CAD build for the part. Positions are in the model's coordinates, mm. Round coordinates to 2 decimals unless told otherwise and drop trailing zeros. Order: outer loops, then holes, each group sorted by start corner. A loop starts at its lowest first (then second) coordinate and runs counter-clockwise, first axis right, second up. Notation, with made-up numbers: M 8.5,73 L 34.5,73 A19 ccw 34.5,86 Z; hole C -4,-17.5 d10. An arc over 180 degrees is marked long. Answer as a JSON object with one key per item and string values.
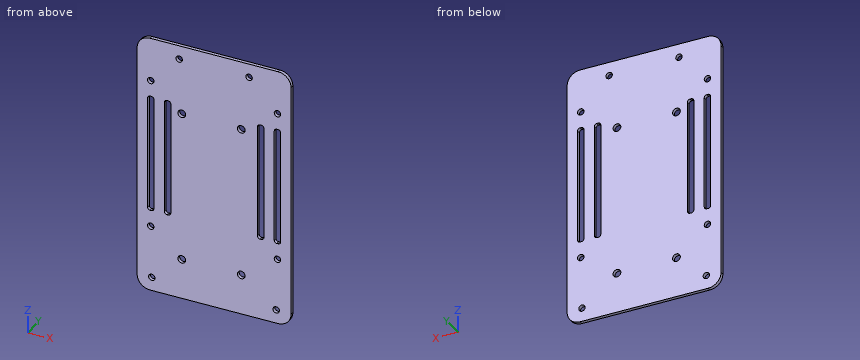
```python
from build123d import *

# Parameters (mm, degrees)
SKETCH2_W           = 59.5
SKETCH2_H           = 100.3
SKETCH2_R           = 1.25
SKETCH2_R_2         = 1.5
BOSS_EXTRUDE1_DEPTH = 1.35
FILLET1_R           = 5
CUT_EXTRUDE1_REACH  = 64.853
SKETCH3_W           = 2.5
SKETCH3_H           = 45.5
FILLET2_R           = 1


with BuildPart() as part:
    # Sketch2 → Boss-Extrude1 (new body)
    with BuildSketch(Plane(origin=(0, 0, 0), x_dir=(1, 0, 0), z_dir=(0, 1, 0))):
        with Locations((0, 5.2)):
            Rectangle(SKETCH2_W, SKETCH2_H)
        with Locations(Location((-24.5, 29.84, 0), (0, 0, 90))):
            Circle(SKETCH2_R, mode=Mode.SUBTRACT)
        with Locations(Location((-24.085, 50.1, 0), (0, 0, 90))):
            Circle(SKETCH2_R, mode=Mode.SUBTRACT)
        with Locations(Location((24.015, 50.1, 0), (0, 0, 90))):
            Circle(SKETCH2_R, mode=Mode.SUBTRACT)
        with Locations(Location((24.5, 29.84, 0), (0, 0, 90))):
            Circle(SKETCH2_R, mode=Mode.SUBTRACT)
        with Locations(Location((24.5, -28.16, 0), (0, 0, 90))):
            Circle(SKETCH2_R, mode=Mode.SUBTRACT)
        with Locations(Location((-24.5, -28.16, 0), (0, 0, 90))):
            Circle(SKETCH2_R, mode=Mode.SUBTRACT)
        with Locations(Location((-13.485, -39.7, 0), (0, 0, 90))):
            Circle(SKETCH2_R, mode=Mode.SUBTRACT)
        with Locations(Location((13.515, -39.7, 0), (0, 0, 90))):
            Circle(SKETCH2_R, mode=Mode.SUBTRACT)
        with Locations(Location((-12.5, -18.16, 0), (0, 0, 90))):
            Circle(SKETCH2_R_2, mode=Mode.SUBTRACT)
        with Locations(Location((10.5, -18.16, 0), (0, 0, 90))):
            Circle(SKETCH2_R_2, mode=Mode.SUBTRACT)
        with Locations(Location((10.5, 39.84, 0), (0, 0, 90))):
            Circle(SKETCH2_R_2, mode=Mode.SUBTRACT)
        with Locations(Location((-12.5, 39.84, 0), (0, 0, 90))):
            Circle(SKETCH2_R_2, mode=Mode.SUBTRACT)
    extrude(amount=BOSS_EXTRUDE1_DEPTH)

    # Fillet1
    fillet1_edges = [part.edges().sort_by_distance(p)[0] for p in [
        (29.75, 0.675, -55.35),
        (29.75, 0.675, 44.95),
        (-29.75, 0.675, 44.95),
        (-29.75, 0.675, -55.35),
    ]]
    fillet(fillet1_edges, radius=FILLET1_R)

    # Sketch3 → Cut-Extrude1 (cut, up to next)
    with BuildSketch(Plane(origin=(0, 1.35, 0), x_dir=(1, 0, 0), z_dir=(0, 1, 0)), mode=Mode.PRIVATE) as cut_extrude1_sk1:
        with Locations((18, 0.84)):
            Rectangle(SKETCH3_W, SKETCH3_H)
    cut_extrude1_tool1 = extrude(cut_extrude1_sk1.sketch, amount=-CUT_EXTRUDE1_REACH, mode=Mode.PRIVATE) & part.part
    # Sketch3 → Cut-Extrude1 (cut, up to next)
    with BuildSketch(Plane(origin=(0, 1.35, 0), x_dir=(1, 0, 0), z_dir=(0, 1, 0)), mode=Mode.PRIVATE) as cut_extrude1_sk2:
        with Locations((-24.5, 0.84)):
            Rectangle(SKETCH3_W, SKETCH3_H)
    cut_extrude1_tool2 = extrude(cut_extrude1_sk2.sketch, amount=-CUT_EXTRUDE1_REACH, mode=Mode.PRIVATE) & part.part
    # Sketch3 → Cut-Extrude1 (cut, up to next)
    with BuildSketch(Plane(origin=(0, 1.35, 0), x_dir=(1, 0, 0), z_dir=(0, 1, 0)), mode=Mode.PRIVATE) as cut_extrude1_sk3:
        with Locations((-18, 0.84)):
            Rectangle(SKETCH3_W, SKETCH3_H)
    cut_extrude1_tool3 = extrude(cut_extrude1_sk3.sketch, amount=-CUT_EXTRUDE1_REACH, mode=Mode.PRIVATE) & part.part
    # Sketch3 → Cut-Extrude1 (cut, up to next)
    with BuildSketch(Plane(origin=(0, 1.35, 0), x_dir=(1, 0, 0), z_dir=(0, 1, 0)), mode=Mode.PRIVATE) as cut_extrude1_sk4:
        with Locations((24.5, 0.84)):
            Rectangle(SKETCH3_W, SKETCH3_H)
    cut_extrude1_tool4 = extrude(cut_extrude1_sk4.sketch, amount=-CUT_EXTRUDE1_REACH, mode=Mode.PRIVATE) & part.part
    add(cut_extrude1_tool1.solids().sort_by_distance((18, 1.35, -0.84))[0], mode=Mode.SUBTRACT)
    add(cut_extrude1_tool2.solids().sort_by_distance((-24.5, 1.35, -0.84))[0], mode=Mode.SUBTRACT)
    add(cut_extrude1_tool3.solids().sort_by_distance((-18, 1.35, -0.84))[0], mode=Mode.SUBTRACT)
    add(cut_extrude1_tool4.solids().sort_by_distance((24.5, 1.35, -0.84))[0], mode=Mode.SUBTRACT)

    # Fillet2
    fillet2_edges = [part.edges().sort_by_distance(p)[0] for p in [
        (-23.25, 0.675, -23.59),
        (-23.25, 0.675, 21.91),
        (-25.75, 0.675, 21.91),
        (-25.75, 0.675, -23.59),
        (-16.75, 0.675, -23.59),
        (-16.75, 0.675, 21.91),
        (-19.25, 0.675, 21.91),
        (-19.25, 0.675, -23.59),
        (19.25, 0.675, -23.59),
        (19.25, 0.675, 21.91),
        (16.75, 0.675, 21.91),
        (16.75, 0.675, -23.59),
        (25.75, 0.675, -23.59),
        (25.75, 0.675, 21.91),
        (23.25, 0.675, 21.91),
        (23.25, 0.675, -23.59),
    ]]
    fillet(fillet2_edges, radius=FILLET2_R)


solid = part.part
```
Item 1: Saw through at D-D on z = 18.16. List the corners of the cut face in (x, y), and give its area (3 significant figures).
Worked answers:
{"outline": "M -29.75,0 L -25.75,0 L -25.75,1.35 L -29.75,1.35 Z; M -23.25,0 L -19.25,0 L -19.25,1.35 L -23.25,1.35 Z; M -16.75,0 L -14,0 L -14,1.35 L -16.75,1.35 Z; M -11,0 L 9,0 L 9,1.35 L -11,1.35 Z; M 12,0 L 16.75,0 L 16.75,1.35 L 12,1.35 Z; M 19.25,0 L 23.25,0 L 23.25,1.35 L 19.25,1.35 Z; M 25.75,0 L 29.75,0 L 29.75,1.35 L 25.75,1.35 Z", "area": "58.7 mm2"}
Item 2: Saw through at A-A on z = -39.84. List the corners of the cut face in (x, y), and give its area (3 significant figures).
Worked answers:
{"outline": "M -29.75,0 L -14,0 L -14,1.35 L -29.75,1.35 Z; M -11,0 L 9,0 L 9,1.35 L -11,1.35 Z; M 12,0 L 29.75,0 L 29.75,1.35 L 12,1.35 Z", "area": "72.2 mm2"}
Item 3: Saw through at C-C on z = -9. List the corners of the cut face in (x, y).
Worked answers:
{"outline": "M -29.75,0 L -25.75,0 L -25.75,1.35 L -29.75,1.35 Z; M -23.25,0 L -19.25,0 L -19.25,1.35 L -23.25,1.35 Z; M -16.75,0 L 16.75,0 L 16.75,1.35 L -16.75,1.35 Z; M 19.25,0 L 23.25,0 L 23.25,1.35 L 19.25,1.35 Z; M 25.75,0 L 29.75,0 L 29.75,1.35 L 25.75,1.35 Z"}
Item 4: Wall check: line 1 along X through (y, z) = (0.7, -6.5); line 2 along X through (y, z) = (0.5, -29.84); line 3 along X through (y, z) = (0.8, -39.84). Give the ranges that are in metal, low to high. Write a range as [from, to].
Worked answers:
{"line 1": "x = [-29.75, -25.75], [-23.25, -19.25], [-16.75, 16.75], [19.25, 23.25], [25.75, 29.75]", "line 2": "x = [-29.75, -25.75], [-23.25, 23.25], [25.75, 29.75]", "line 3": "x = [-29.75, -14], [-11, 9], [12, 29.75]"}
Item 5: Saw through at B-B on x = 10.5. List the corners of the cut face in (y, z), and give its area (3 significant figures).
Worked answers:
{"outline": "M 0,-55.35 L 1.35,-55.35 L 1.35,-41.34 L 0,-41.34 Z; M 0,-38.34 L 1.35,-38.34 L 1.35,16.66 L 0,16.66 Z; M 0,19.66 L 1.35,19.66 L 1.35,44.95 L 0,44.95 Z", "area": "127 mm2"}
